```python
from build123d import *

# Parameters (mm, degrees)
SKETCH_1_W             = 9.1
SKETCH_1_H             = 7.1
SKETCH_1_W_2           = 7.5
SKETCH_1_H_2           = 5.5
EXTRUDE_1_DEPTH        = 7.2
SKETCH_1_3_W           = 1.05
SKETCH_1_3_H           = 5.5
EXTRUDE_2_DEPTH        = 5
SKETCH_1_4_W           = 9.1
SKETCH_1_4_H           = 7.1
EXTRUDE_3_DEPTH        = 0.6
EXTRUDE_4_DEPTH        = 5
EXTRUDE_START          = -0.6
EXTRUDE_5_DEPTH        = 0.6
SKETCH_2_W             = 1.05
SKETCH_2_H             = 1
CUT_EXTRUDE_1_DEPTH    = 7.1
SKETCH_4_W             = 4
SKETCH_4_H             = 1.5
EXTRUDE_7_DEPTH        = 6
SKETCH_5_R             = 1
CUT_EXTRUDE_2_DEPTH    = 1.5
PATTERN_LINEAR_2_COUNT = 2
PATTERN_LINEAR_2_PITCH = 13.1


with BuildPart() as part:
    # Sketch 1 → Extrude 1 (new body)
    with BuildSketch(Plane(origin=(0, 0, 0), x_dir=(1, 0, 0), z_dir=(0, 1, 0))):
        Rectangle(SKETCH_1_W, SKETCH_1_H)
        Rectangle(SKETCH_1_W_2, SKETCH_1_H_2, mode=Mode.SUBTRACT)
    extrude(amount=EXTRUDE_1_DEPTH)

    # Sketch 1_3 → Extrude 2 (add)
    with BuildSketch(Plane(origin=(0, 0, 0), x_dir=(1, 0, 0), z_dir=(0, 1, 0))):
        with Locations((-3.225, 0)):
            Rectangle(SKETCH_1_3_W, SKETCH_1_3_H)
        with Locations((3.225, 0)):
            Rectangle(SKETCH_1_3_W, SKETCH_1_3_H)
    extrude(amount=EXTRUDE_2_DEPTH)

    # Sketch 1_4 → Extrude 3 (add)
    with BuildSketch(Plane(origin=(0, 0, 0), x_dir=(1, 0, 0), z_dir=(0, 1, 0))):
        Rectangle(SKETCH_1_4_W, SKETCH_1_4_H)
    extrude(amount=-EXTRUDE_3_DEPTH)

    # Sketch 1_5 → Extrude 4 (add)
    with BuildSketch(Plane(origin=(0, 0, 0), x_dir=(1, 0, 0), z_dir=(0, 1, 0))):
        with BuildLine():
            Line((4.55, 3.55), (4.55, 2.75))
            Line((4.55, 2.75), (5.85, 2.75))
            ThreePointArc((5.85, 2.75), (8.6, 0), (5.85, -2.75))
            Line((5.85, -2.75), (4.55, -2.75))
            Line((4.55, -2.75), (4.55, -3.55))
            Line((4.55, -3.55), (5.85, -3.55))
            ThreePointArc((5.85, -3.55), (9.4, 0), (5.85, 3.55))
            Line((5.85, 3.55), (4.55, 3.55))
        make_face()
    extrude(amount=EXTRUDE_4_DEPTH)

    # Sketch 1_6 → Extrude 5 (add)
    with BuildSketch(Plane(origin=(0, 0, 0), x_dir=(1, 0, 0), z_dir=(0, 1, 0)).offset(EXTRUDE_START)):
        with BuildLine():
            Line((5.85, 2.75), (4.55, 2.75))
            Line((4.55, 2.75), (4.55, -2.75))
            Line((4.55, -2.75), (5.85, -2.75))
            ThreePointArc((5.85, -2.75), (8.6, 0), (5.85, 2.75))
        make_face()
        with BuildLine():
            Line((4.55, 3.55), (4.55, 2.75))
            Line((4.55, 2.75), (5.85, 2.75))
            ThreePointArc((5.85, 2.75), (8.6, 0), (5.85, -2.75))
            Line((5.85, -2.75), (4.55, -2.75))
            Line((4.55, -2.75), (4.55, -3.55))
            Line((4.55, -3.55), (5.85, -3.55))
            ThreePointArc((5.85, -3.55), (9.4, 0), (5.85, 3.55))
            Line((5.85, 3.55), (4.55, 3.55))
        make_face()
    extrude(amount=EXTRUDE_5_DEPTH)

    # Sketch 2 → Cut-Extrude 1 (cut)
    with BuildSketch(Plane(origin=(0, 0, -3.55), x_dir=(-1, 0, 0), z_dir=(0, 0, -1))):
        with Locations((-2.225, 6.7)):
            Rectangle(SKETCH_2_W, SKETCH_2_H)
    extrude(amount=-CUT_EXTRUDE_1_DEPTH, mode=Mode.SUBTRACT)

    # Sketch 4 → Extrude 7 (add)
    with BuildSketch(Plane.XY.offset(3.55)):
        with Locations((0, 0.15)):
            Rectangle(SKETCH_4_W, SKETCH_4_H)
    extrude_7 = extrude(amount=EXTRUDE_7_DEPTH)

    # Sketch 5 → Cut-Extrude 2 (cut)
    with BuildSketch(Plane(origin=(0, 0.9, 0), x_dir=(1, 0, 0), z_dir=(0, 1, 0))):
        with Locations(Location((0, -5.05, 0), (0, 0, 180))):
            Circle(SKETCH_5_R)
        with Locations(Location((0, -7.85, 0), (0, 0, 180))):
            Circle(SKETCH_5_R)
    cut_extrude_2 = extrude(amount=-CUT_EXTRUDE_2_DEPTH, mode=Mode.SUBTRACT)

    # Pattern Linear 2: Extrude 7, Cut-Extrude 2 ×2
    with Locations(*[(0, 0, -i * PATTERN_LINEAR_2_PITCH) for i in range(1, PATTERN_LINEAR_2_COUNT)]):
        add(extrude_7)
        add(cut_extrude_2, mode=Mode.SUBTRACT)


solid = part.part
```
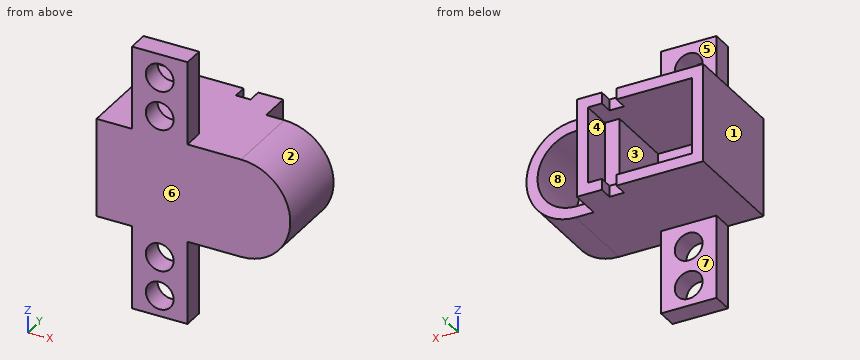
The listing builds one solid part. Answer for the finished solid, in the listing's coordinates (mm). Face numbers are marked on the shaded views. A direction names the side the tool comes from. Coordinates: 2 decimals unless noted, no trailing zeros. Loops run counter-clockwise (first coordinate to the right, second up) from the corner with the lowest first, then second, coordinate; pieces in that order, holes last. Notation, with made-up numbers: M 21,47.5 L 25,47.5 A27 ccw 25,85.5 Z; hole C -29.75,-32 d9. An arc over 180 degrees is marked long. Answer as a JSON object with one key per item and string values. Group by question number.
Item 1: Section A-A (z = -8.05) is taken. Write down the section's boundary in (x, y), and give its area (3 significant figures).
Item 2: Section B-B (y = 4.5) is taken. Write down the section's boundary in (x, z), and give its area (3 significant figures).
Item 3: Determine the mould class of the marked faces 1, 2, 3 and 4 for opening direction Z: +Z half, -Z half, draft (parallel to the pull), parting line (faces both ways), or undercut.
Item 4: Consider L1, parallel to Z at x = 0, y = 0.6; L2, parallel to Z at x = 1.25, y = 0.25; L3, parallel to Z at x = 0, y = -0.15. Determine where each line is inside the solid, lowest interval first.
Item 5: Section D-D (y = 0.5) is taken. Write down the section's boundary in (x, z).
Item 6: Section C-C (x = 0) is taken. Write down the section's boundary in (y, z).
Item 7: Which of the six approach directions +Z, -Z, +X, -X, +Y, -Y give full straight-line access (tool end or side, diameter ignored) to the marked faces 5, 6, 7 and 8?
Item 8: Each of these flat-tipped pins is pushed along its axis until it touches: P1, Ø1.2, axis at x = -3.5, z = 1, coming from the +Y side; P2, Ø2.5, axis at x = 2, y = 3, coming from the +Z side; P3, Ø2.5, axis at y = 6.5, z = 0.5, coming from the +X side; P4, Ø4, axis at x = 5.5, y = 4.5, coming from the -Z side. Where does it stop, or does it pass through?
Solved:
{
 "1": {"outline": "M -2,-0.6 L -1,-0.6 L -1,0.9 L -2,0.9 Z; M 1,-0.6 L 2,-0.6 L 2,0.9 L 1,0.9 Z", "area": "3.00 mm2"},
 "2": {"outline": "M -4.55,-3.55 L 5.85,-3.55 A3.55 ccw 5.85,3.55 L -4.55,3.55 Z; hole M -2.7,-2.75 L 2.7,-2.75 L 2.7,2.75 L -2.7,2.75 Z; hole M 4.55,-2.75 L 5.85,-2.75 A2.75 ccw 5.85,2.75 L 4.55,2.75 Z", "area": "44.9 mm2"},
 "3": {"face 1": "draft", "face 2": "parting line", "face 3": "undercut", "face 4": "undercut"},
 "4": {"L1": "z = -9.55 to -9.05, -7.05 to -6.25, -4.25 to -2.75, 2.75 to 4.05, 6.05 to 6.85, 8.85 to 9.55", "L2": "z = -9.55 to -2.75, 2.75 to 9.55", "L3": "z = -9.55 to -9.05, -7.05 to -6.25, -4.25 to 4.05, 6.05 to 6.85, 8.85 to 9.55"},
 "5": {"outline": "M -4.55,-3.55 L -2,-3.55 L -2,-9.55 L 2,-9.55 L 2,-3.55 L 5.85,-3.55 A3.55 ccw 5.85,3.55 L 2,3.55 L 2,9.55 L -2,9.55 L -2,3.55 L -4.55,3.55 Z; hole M -2.7,-2.75 L 2.7,-2.75 L 2.7,2.75 L -2.7,2.75 Z; hole C 0,-8.05 d2; hole C 0,-5.25 d2; hole C 0,5.05 d2; hole C 0,7.85 d2; hole M 4.55,-2.75 L 5.85,-2.75 A2.75 ccw 5.85,2.75 L 4.55,2.75 Z"},
 "6": {"outline": "M -0.6,-9.55 L 0.9,-9.55 L 0.9,-9.05 L -0.6,-9.05 Z; M -0.6,-7.05 L 0.9,-7.05 L 0.9,-6.25 L -0.6,-6.25 Z; M -0.6,-4.25 L 0.9,-4.25 L 0.9,-3.55 L 7.2,-3.55 L 7.2,-2.75 L 0,-2.75 L 0,2.75 L 7.2,2.75 L 7.2,3.55 L 0.9,3.55 L 0.9,4.05 L -0.6,4.05 Z; M -0.6,6.05 L 0.9,6.05 L 0.9,6.85 L -0.6,6.85 Z; M -0.6,8.85 L 0.9,8.85 L 0.9,9.55 L -0.6,9.55 Z"},
 "7": {"face 5": "+Z, +X, -X, +Y", "face 6": "+Z, -Z, +X, -X, -Y", "face 7": "-Z, +X, -X, +Y", "face 8": "+Y"},
 "8": {"P1": "stops at y = 7.2", "P2": "stops at z = 3.55", "P3": "stops at x = 4.55", "P4": "stops at z = -3.55"}
}
